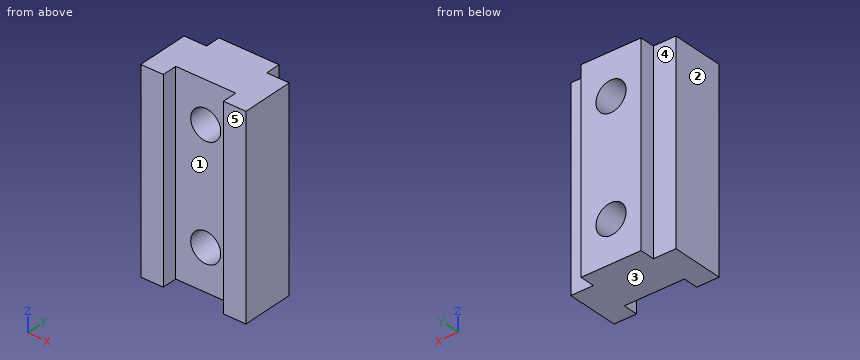
```python
from build123d import *

# Parameters (mm, degrees)
F1_DEPTH = 25.4
F2_DEPTH = 139.7
F3_R     = 12.7
F4_DEPTH = 44.45
F5_DEPTH = 44.45


with BuildPart() as f1:
    # F0 (on Top) → F1 (new body)
    with BuildSketch(Plane.XY):
        Polygon((-19.05, 0), (0, 0), (0, 12.7), (50.8, 12.7), (50.8, 0), (69.85, 0), (69.85, 44.45), (50.8, 44.45), (50.8, 57.15), (0, 57.15), (0, 44.45), (-19.05, 44.45), align=None)
    extrude(amount=F1_DEPTH)

    # F1_face (on face) → F2 (join)
    with BuildSketch(Plane(origin=(25.4, 29.482143, 25.4), x_dir=(1, 0, 0), z_dir=(0, 0, 1))):
        Polygon((-44.45, -29.482143), (-25.4, -29.482143), (-25.4, -16.782143), (25.4, -16.782143), (25.4, -29.482143), (44.45, -29.482143), (44.45, 14.967857), (25.4, 14.967857), (25.4, 27.667857), (-25.4, 27.667857), (-25.4, 14.967857), (-44.45, 14.967857), align=None)
    extrude(amount=F2_DEPTH)

    # F3 (on face) → F4 (cut, through all)
    with BuildSketch(Plane(origin=(0, 57.15, 0), x_dir=(-1, 0, 0), z_dir=(0, 1, 0))):
        with Locations((-25.4, 130.175)):
            Circle(F3_R)
    extrude(amount=-F4_DEPTH, mode=Mode.SUBTRACT)

    # F3 (on face) → F5 (cut, through all)
    with BuildSketch(Plane(origin=(0, 57.15, 0), x_dir=(-1, 0, 0), z_dir=(0, 1, 0))):
        with Locations((-25.4, 34.925)):
            Circle(F3_R)
    extrude(amount=-F5_DEPTH, mode=Mode.SUBTRACT)


solid = f1.part
```
Part model, mm, in its own coordinate system. Face numbers are marked on the shaded views. A direction names the side the tool comes from. Give positions to 0.01 mm unless a question says otherwise; leave off trailing zeros. Order: outer loops, then holes, each group sorted by start corner. A loop starts at its lowest first (then second) coordinate and runs counter-clockwise, first axis right, second up. Notation, with made-up numbers: M 22.5,-19 L 81.5,-19 A33 cw 81.5,10 Z; hole C 37.5,-24 d4. An arc over 180 degrees is marked long. Use a Markdown table: item, result. Add a question column.
(1) Saw through at D-D, the plane z = 65.5. Give the cut face in (x, y).
(2) Saw through at B-B, the plane y = 4.5. Give the cut face in (x, z), and give its area (3 significant figures).
(3) Saw through at C-C, the plane z = 138. Give the cut face in (x, y), and give its area (3 significant figures).
(4) 3-axis set-ups, long thin cutter, end or side, ignore diameter. For the marked faces 4 and 5: which of +Z, -Z, +X, -X, +Y, -Y reach the whole face in a straight line?
(5) Saw through at A-A, the plane x = 25.4. Give the cut face in (y, z) (3 decimals), and give its area (3 significant figures).
(6) Mould opens along X. For the marked faces 1, 2 and 3 say: +X half, -X half, draft (parallel to the pull), parting line (faces both ways), or undercut.
(7) Probe line 1 along Z through (x, y) = (25.4, 33) (3 decimals); line 2 along X through (y, z) = (4, 42). List the from-to ranges inside material, lowest first. Write a range as [from, to].
(8) Drop flat-ended pins along their axis: P1, Ø21, axis at x = -13, z = 114, coming from the +Y side; P2, Ø6.5, axis at y = 50, z = 68, coming from the +X side. Give the stop position or say it passes through.
Answer key:
| question | item | result |
|---|---|---|
| 1 | outline | M -19.05,0 L 0,0 L 0,12.7 L 50.8,12.7 L 50.8,0 L 69.85,0 L 69.85,44.45 L 50.8,44.45 L 50.8,57.15 L 0,57.15 L 0,44.45 L -19.05,44.45 Z |
| 2 | outline | M -19.05,0 L 0,0 L 0,165.1 L -19.05,165.1 Z; M 50.8,0 L 69.85,0 L 69.85,165.1 L 50.8,165.1 Z |
| 2 | area | 6,290 mm^2 |
| 3 | outline | M -19.05,0 L 0,0 L 0,12.7 L 15.4,12.7 L 15.4,57.15 L 0,57.15 L 0,44.45 L -19.05,44.45 Z; M 35.4,12.7 L 50.8,12.7 L 50.8,0 L 69.85,0 L 69.85,44.45 L 50.8,44.45 L 50.8,57.15 L 35.4,57.15 Z |
| 3 | area | 3,060 mm^2 |
| 4 | face 4 | +Z, -Z, -X, +Y |
| 4 | face 5 | +Z, -Z, +X, -X, -Y |
| 5 | outline | M 12.7,0 L 57.15,0 L 57.15,22.225 L 12.7,22.225 Z; M 12.7,47.625 L 57.15,47.625 L 57.15,117.475 L 12.7,117.475 Z; M 12.7,142.875 L 57.15,142.875 L 57.15,165.1 L 12.7,165.1 Z |
| 5 | area | 5,080 mm^2 |
| 6 | face 1 | undercut |
| 6 | face 2 | -X half |
| 6 | face 3 | draft |
| 7 | line 1 | [0, 22.225], [47.625, 117.475], [142.875, 165.1] |
| 7 | line 2 | [-19.05, 0], [50.8, 69.85] |
| 8 | P1 | y = 44.45 |
| 8 | P2 | x = 50.8 |
